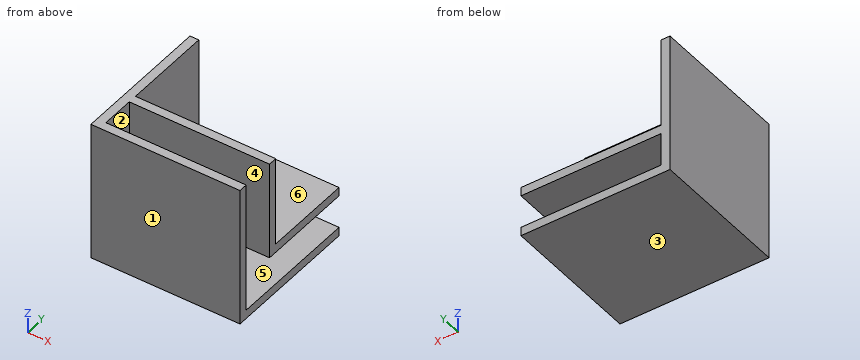
Autodesk Inventor part; units mm, degrees
ref_plane "YZ Plane" through (0, 0, 0) normal (1, 0, 0) x (0, 1, 0)
ref_plane "XZ Plane" through (0, 0, 0) normal (0, 1, 0) x (-1, 0, 0)
ref_plane "XY Plane" through (0, 0, 0) normal (0, 0, 1) x (1, 0, 0)
sketch "Sketch3" plane through (0, 0, 0) normal (1, 0, 0) x (0, 1, 0)
  line L0 (0, 0) -> (25.4, 0)
  line L1 (25.4, 0) -> (25.4, -25.4)
  line L2 (25.4, -25.4) -> (0, -25.4)
  line L3 (0, -25.4) -> (0, 0)
  line L4 (25.4, -23.8125) -> (1.5875, -23.8125)
  line L5 (1.5875, -23.8125) -> (1.5875, 0)
  line L6 (7.5819, -17.8125) -> (25.4, -17.8125)
  line L7 (7.5819, 0) -> (7.5819, -17.8125)
  line L8 (9.1694, 1) -> (9.1694, -16.225)
  line L9 (9.1694, -16.225) -> (25.4, -16.225)
  point P0 (25.4, -16.225)
  point P1 (9.1694, 0)
  dimension "d15" = 25.4
  dimension "d16" = 25.4
  dimension "d17" = 1.5875
  dimension "d18" = 6
  dimension "d19" = 1.5875
  dimension "d24" = 5.9944
extrude "Extrusion3" add sketch "Sketch3" along normal blind 25.4 contours L0 L5 L4 L1 L2 L3 | L0 L8 L9 L1 L6 L7
sketch "Sketch4" plane through (0, 0, 0) normal (-1, 0, 0) x (0, 0, 1)
  line L0 (-25.4, 0) -> (-25.4, 25.4)
  line L1 (-25.4, 25.4) -> (0, 25.4)
  line L2 (0, 25.4) -> (0, 0)
  line L3 (0, 0) -> (-25.4, 0)
  line L4 (-25.4, 0) -> (-25.4, 25.4)
extrude "Extrusion4" add sketch "Sketch4" along normal blind 1.5875
properties part number "clip corner"
CAD build for the part. Positions are in the model's coordinates, mm. Face numbers are marked on the shaded views. A direction names the side the tool comes from. Round coordinates to 2 decimals unless told otherwise and drop trailing zeros. Order: outer loops, then holes, each group sorted by start corner. A loop starts at its lowest first (then second) coordinate and runs counter-clockwise, first axis right, second up. Notation, with made-up numbers: (71.5, 69) -> (120.5, 69) arc R18 cw to (120.5, 97) -> close; hole circle Ø6 at (86, 78.5). An arc over 180 degrees is marked (long way). Write item = value, one per line. Start each with the question number.
(1) Probe line 1 (Z direction, x = 15.75, y = 13.5) (1 decimal); line 2 (Y direction, x = 18.5, z = -12.5); line 3 (Z direction, x = 16.75, y = 8.5). List the from-to ranges inside material, lowest first. Write a range as [from, to].
(2) Cut at D-D, the plane z = -12.5. List the corners of the cut face in (x, y).
(3) Cut at B-B, the plane z = -21. List the corners of the cut face in (x, y).
(4) Pull direction Y, two halves, no side cores. Call the marked faces 1, 2 and 3: released by +Y, released by -Y, zero draft, split by the parting line, or undercut.
(5) Which spindle directions (+Z, -Z, +X, -X, +Y, -Y) get a long thin tool onto all of the face, cutting with end or side? Do the marked faces 4, 5 and 6. Say none if no direction does.
(6) Pin check, flat tips, straight feed: P1, Ø10, axis at y = 10, z = -12, coming from the +X side; P2, Ø1, axis at x = 8, y = 13, coming from the +Z side (3 decimals); P3, Ø7, axis at y = 17.5, z = -7.5, coming from the +X side; P4, Ø5, axis at x = 11, z = -8.5, coming from the +Y side. Stop position of each tip, or through.
(7) Cut at A-A, the plane x = 22. List the corners of the cut face in (y, z) (1 decimal).
(8) Cut at C-C, the plane y = 23. List the corners of the cut face in (x, z) (1 decimal), then the cut area to 3 significant figures.
Model answer:
q1.line_1 = [-25.4, -23.8], [-17.8, -16.2]
q1.line_2 = [0, 1.59], [7.58, 9.17]
q1.line_3 = [-25.4, -23.81], [-17.81, 0]
q2.outline = (-1.59, 0) -> (25.4, 0) -> (25.4, 1.59) -> (0, 1.59) -> (0, 7.58) -> (25.4, 7.58) -> (25.4, 9.17) -> (0, 9.17) -> (0, 25.4) -> (-1.59, 25.4) -> close
q3.outline = (-1.59, 0) -> (25.4, 0) -> (25.4, 1.59) -> (0, 1.59) -> (0, 25.4) -> (-1.59, 25.4) -> close
q4.face_1 = released by -Y
q4.face_2 = undercut
q4.face_3 = zero draft
q5.face_4 = +Z, +X
q5.face_5 = +X, +Y
q5.face_6 = +Z, +X, +Y
q6.P1 = 25.4
q6.P2 = -16.225
q6.P3 = 0
q6.P4 = 9.17
q7.outline = (0, -25.4) -> (25.4, -25.4) -> (25.4, -23.8) -> (1.6, -23.8) -> (1.6, 0) -> (0, 0) -> close; (7.6, -17.8) -> (25.4, -17.8) -> (25.4, -16.2) -> (9.2, -16.2) -> (9.2, 0) -> (7.6, 0) -> close
q8.outline = (-1.6, -25.4) -> (25.4, -25.4) -> (25.4, -23.8) -> (0, -23.8) -> (0, -17.8) -> (25.4, -17.8) -> (25.4, -16.2) -> (0, -16.2) -> (0, 0) -> (-1.6, 0) -> close
q8.area = 121 mm2
